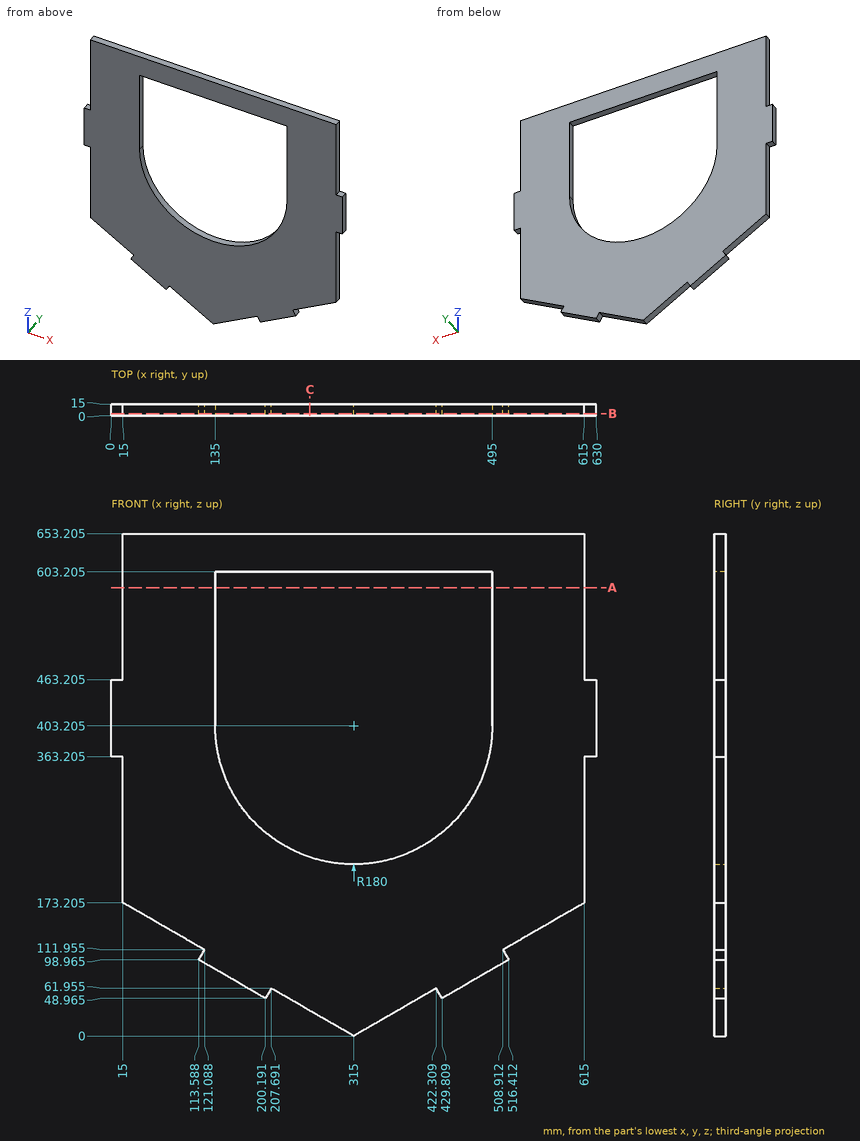
Study the drawing (mm; zero at the part's minimum x, y, z) and answer. Coordinates: 2 decimals unless noted, no trailing zeros. Write each loop counter-clockwise with the first axis right and the second up, starting at its lowest first coordinate (ties: lowest second). Pieces come first, ordered by that corner, then holes.
Q1. A cutting plane is placed at A-A, the plane z = 583. Give the vertices of the cut face in (x, y).
Q2. Each of these flat-tipped pins is pushed along its axis until it touches: pin 1 Ø4.5 at (x, y) = (394, 5.5) entering from -Z; pin 2 Ø1.5 at (y, z) = (11, 131.5) entering from -X (1 decimal); pin 3 Ø7.5 at (x, y) = (9, 7) entering from -Z (3 decimals); pin 4 Ø5 at (x, z) = (84, 249) entering from -Y. Where does it stop, or does it pass through?
Q3. Find the intervals of material crossed by line 1 (X direction, y = 14.25, z = 449.5); line 2 (X direction, y = 12, z = 508); line 3 (Z direction, x = 213, y = 7.5) (1 decimal), in increasing order.
Q4. A cutting plane is placed at B-B, the plane y = 2.5. Give the vertices of the cut face in (x, z) (1 decimal).
Q5. A cutting plane is placed at C-C, the plane x = 258. Give the vertices of the cut face in (y, z) (1 decimal).
Findings below:
1. outline: (15, 0) - (135, 0) - (135, 15) - (15, 15) - close; (495, 0) - (615, 0) - (615, 15) - (495, 15) - close
2. pin 1: stops at z = 44.31
2. pin 2: stops at x = 85.9
2. pin 3: stops at z = 363.205
2. pin 4: stops at y = 0
3. line 1: x = 0 to 135, 495 to 630
3. line 2: x = 15 to 135, 495 to 615
3. line 3: z = 58.9 to 254.9, 603.2 to 653.2
4. outline: (0, 363.2) - (15, 363.2) - (15, 173.2) - (121.1, 112) - (113.6, 99) - (200.2, 49) - (207.7, 62) - (315, 0) - (422.3, 62) - (429.8, 49) - (516.4, 99) - (508.9, 112) - (615, 173.2) - (615, 363.2) - (630, 363.2) - (630, 463.2) - (615, 463.2) - (615, 653.2) - (15, 653.2) - (15, 463.2) - (0, 463.2) - close; hole (135, 403.2) arc R180 ccw to (495, 403.2) - (495, 603.2) - (135, 603.2) - close
5. outline: (0, 32.9) - (15, 32.9) - (15, 232.5) - (0, 232.5) - close; (0, 603.2) - (15, 603.2) - (15, 653.2) - (0, 653.2) - close
